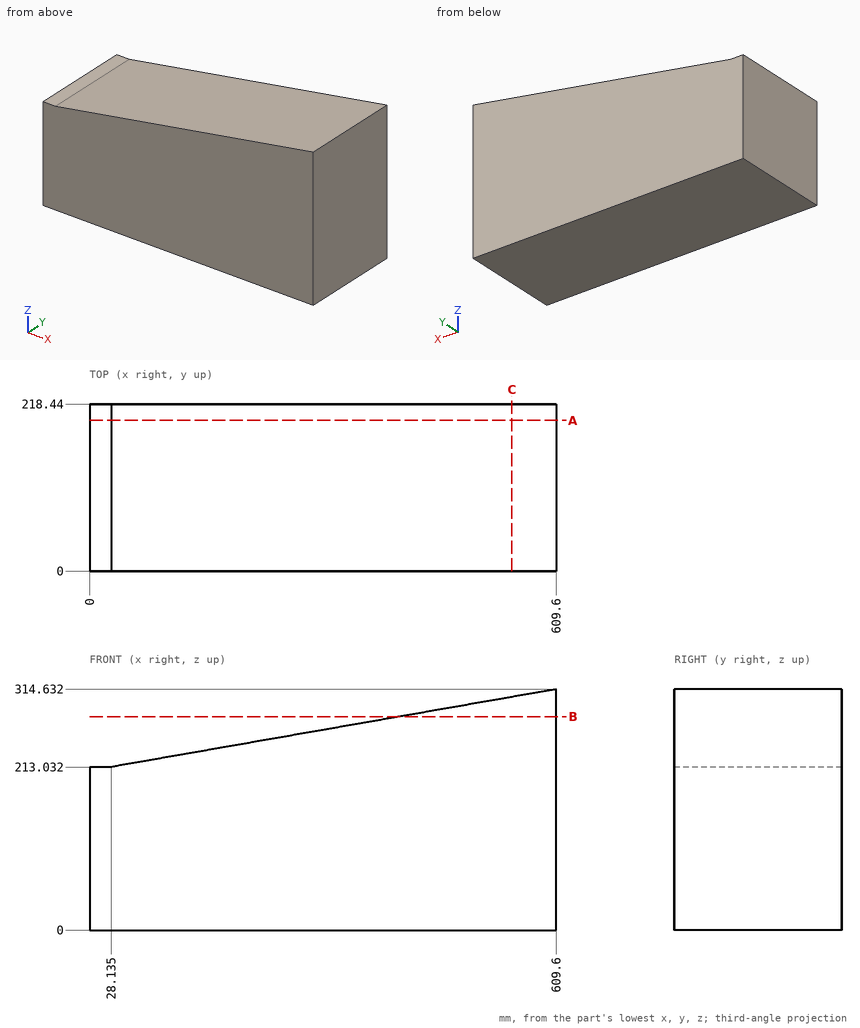
Drawing for the job (mm, zero at the part's lowest x, y, z). Round coordinates to 2 decimals unless told otherwise and drop trailing zeros. Write each loop counter-clockwise with the first axis right and the second up, starting at its lowest first coordinate (ties: lowest second). Pieces come first, ordered by that corner, then holes. Notation, with made-up numbers: M 60.25,-16.5 L 88.25,-16.5 A30 cw 88.25,9.5 Z; hole C 36.5,-23.75 d10. An arc over 180 degrees is marked long. Put each result on its own line as item: value.
Item 1: Cut at C-C (x = 551.5). List the corners of the cut face in (y, z).
Responses:
outline: M 0,0 L 218.44,0 L 218.44,304.48 L 0,304.48 Z
Item 2: Probe L1, parallel to Z at x = 376.5, y = 142; L2, parallel to Z at x = 534.5, y = 81.5. List the from-to ranges inside material, lowest first. Write a range as from..to.
Responses:
L1: 0..273.9
L2: 0..301.51
Item 3: Cut at A-A (y = 197). List the corners of the cut face in (x, z) (1 decimal), and give its area (3 significant figures).
Responses:
outline: M 0,0 L 609.6,0 L 609.6,314.6 L 28.1,213 L 0,213 Z
area: 159,000 mm²
Item 4: Flat gauge pin, fed straight in: P1, Ø8, axis at x = 230, z = 53, coming from the -Y side. Where does the tip first touch, or does it go through?
Responses:
P1: y = 0
Item 5: Cut at B-B (z = 279). List the corners of the cut face in (x, y), and give its area (3 significant figures).
Responses:
outline: M 405.67,0 L 609.6,0 L 609.6,218.44 L 405.67,218.44 Z
area: 44,500 mm²
